from build123d import *

# Parameters (mm, degrees)
BOSS_EXTRUDE1_DEPTH = 243.84
SKETCH2_R           = 2.1828125
CUT_EXTRUDE1_DEPTH  = 2.54
SKETCH3_R           = 2.1828125
CUT_EXTRUDE2_DEPTH  = 246.205601499


with BuildPart() as part:
    # Sketch1 → Boss-Extrude1 (new body)
    with BuildSketch(Plane(origin=(0, 0, 0), x_dir=(1, 0, 0), z_dir=(0, 1, 0))):
        Polygon((0, 0), (0, 19.05), (1.5875, 19.05), (1.5875, 1.5875), (19.05, 1.5875), (19.05, 0), align=None)
    extrude(amount=BOSS_EXTRUDE1_DEPTH)

    # Sketch2 → Cut-Extrude1 (cut)
    with BuildSketch(Plane.XY):
        with Locations((10.16, 233.68)):
            Circle(SKETCH2_R)
        with Locations((10.16, 10.16)):
            Circle(SKETCH2_R)
    extrude(amount=-CUT_EXTRUDE1_DEPTH, mode=Mode.SUBTRACT)

    # Sketch3 → Cut-Extrude2 (cut, through all)
    with BuildSketch(Plane(origin=(1.5875, 0, 0), x_dir=(0, 0, -1), z_dir=(1, 0, 0))):
        with Locations((10.16, 233.68)):
            Circle(SKETCH3_R)
        with Locations((10.16, 10.16)):
            Circle(SKETCH3_R)
    extrude(amount=-CUT_EXTRUDE2_DEPTH, mode=Mode.SUBTRACT)


solid = part.part
Could you check a few things on this model? Use its own coordinates, in mm. A direction names the side the tool comes from. Give positions to 0.01 mm unless a question says otherwise; leave off trailing zeros. Order: outer loops, then holes, each group sorted by start corner. A loop starts at its lowest first (then second) coordinate and runs counter-clockwise, first axis right, second up. Notation, with made-up numbers: (8.5, 4.25) - (19.5, 4.25) arc R23 ccw to (19.5, 24.25) - close; hole circle Ø11 at (41.25, 38). An arc over 180 degrees is marked (long way). One line per item, written item: value. Start each with the question number.
1. Imagine slicing it at D-D on y = 174.5. List the corners of the cut face in (x, z) for me, plus the area to 3 significant figures.
2. If I drill on probe 1 along Y at (x, z) = (0.85, -10.16); probe 2 along X at (y, z) = (233.68, -1.1); probe 3 along Z at (x, y) = (1, 233.68), over which ranges is the centre line in solid material (lowest first)?
3. Imagine slicing it at C-C on z = -10.16. List the corners of the cut face in (x, y) for me, plus the area to 3 significant figures.
4. Thinking about a two-plate mould opening in Z: for faces 3 (the face through (0.8, 231.55, -9.69)), 4 (the face through (5, 243.84, -1)), 5 (the face through (10, 120, -1.588)), which applies, +Z half, -Z half, draft (parallel to the pull), parting line (faces both ways), or undercut?
5. Imagine slicing it at A-A on x = 10.16. List the corners of the cut face in (y, z) for me.
6. For faces 1 (the face through (1.588, 120, -10)), 2 (the face through (12.24, 10.82, -0.78)), which set-ups out of +Z, -Z, +X, -X, +Y, -Y let a thin tool reach every point of the face, with its end or its side?
7. For P1, Ø3.5, axis at y = 233.68, z = -10.16, coming from the +X side; P2, Ø5, axis at y = 148.5, z = -14, coming from the +X side, each with a flat end and sliding along its axis, tell me the tip position at first contact or that it passes through.
8. Imagine slicing it at B-B on y = 10.16. List the corners of the cut face in (x, z) for me, plus the area to 3 significant figures.
Values:
1. outline: (0, -19.05) - (1.59, -19.05) - (1.59, -1.59) - (19.05, -1.59) - (19.05, 0) - (0, 0) - close
1. area: 58.0 mm²
2. probe 1: 0 to 7.98, 12.34 to 231.5, 235.86 to 243.84
2. probe 2: 0 to 7.98, 12.34 to 19.05
2. probe 3: -19.05 to -12.34, -7.98 to 0
3. outline: (0, 0) - (1.59, 0) - (1.59, 7.98) - (0, 7.98) - close; (0, 12.34) - (1.59, 12.34) - (1.59, 231.5) - (0, 231.5) - close; (0, 235.86) - (1.59, 235.86) - (1.59, 243.84) - (0, 243.84) - close
3. area: 373 mm²
4. face 3: undercut
4. face 4: draft
4. face 5: -Z half
5. outline: (0, -1.59) - (7.98, -1.59) - (7.98, 0) - (0, 0) - close; (12.34, -1.59) - (231.5, -1.59) - (231.5, 0) - (12.34, 0) - close; (235.86, -1.59) - (243.84, -1.59) - (243.84, 0) - (235.86, 0) - close
6. face 1: -Z, +X, +Y, -Y
6. face 2: +Z, -Z
7. P1: through
7. P2: x = 1.59
8. outline: (0, -19.05) - (1.59, -19.05) - (1.59, -12.34) - (0, -12.34) - close; (0, -7.98) - (1.59, -7.98) - (1.59, -1.59) - (7.98, -1.59) - (7.98, 0) - (0, 0) - close; (12.34, -1.59) - (19.05, -1.59) - (19.05, 0) - (12.34, 0) - close
8. area: 44.1 mm²
